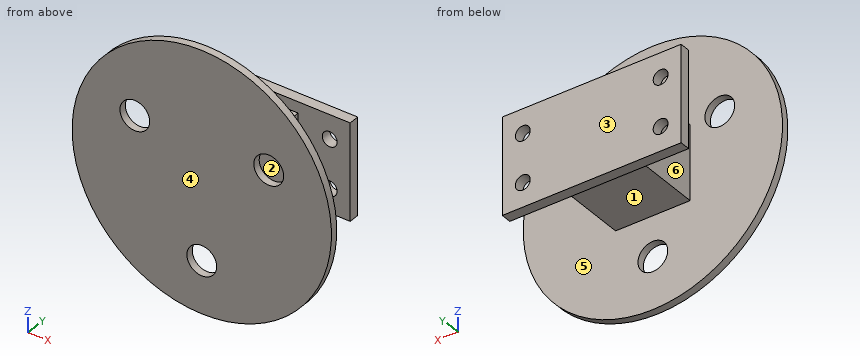
```python
from build123d import *

# Parameters (mm, degrees)
SKETCH1_R           = 87
SKETCH1_R_2         = 10
BOSS_EXTRUDE1_DEPTH = 5
SKETCH2_W           = 50
SKETCH2_H           = 50
BOSS_EXTRUDE2_DEPTH = 50
SKETCH3_W           = 120
SKETCH3_H           = 65
SKETCH3_R           = 5
BOSS_EXTRUDE3_DEPTH = 7


with BuildPart() as part:
    # Sketch1 → Boss-Extrude1 (new body)
    with BuildSketch(Plane(origin=(0, 0, 0), x_dir=(1, 0, 0), z_dir=(0, 1, 0))):
        with Locations(Location((0, 0, 0), (0, 0, 270))):
            Circle(SKETCH1_R)
        with Locations(Location((0, 51.875, 0), (0, 0, 270))):
            Circle(SKETCH1_R_2, mode=Mode.SUBTRACT)
        with Locations(Location((44.926567821, -25.936633975, 0), (0, 0, 270))):
            Circle(SKETCH1_R_2, mode=Mode.SUBTRACT)
        with Locations(Location((-44.923567821, -25.938366025, 0), (0, 0, 270))):
            Circle(SKETCH1_R_2, mode=Mode.SUBTRACT)
    extrude(amount=BOSS_EXTRUDE1_DEPTH)

    # Sketch2 → Boss-Extrude2 (add)
    with BuildSketch(Plane(origin=(0, 5, 0), x_dir=(1, 0, 0), z_dir=(0, 1, 0))):
        Rectangle(SKETCH2_W, SKETCH2_H)
    extrude(amount=BOSS_EXTRUDE2_DEPTH)

    # Sketch3 → Boss-Extrude3 (add)
    with BuildSketch(Plane(origin=(0, 55, 0), x_dir=(1, 0, 0), z_dir=(0, 1, 0))):
        Rectangle(SKETCH3_W, SKETCH3_H)
        with Locations(Location((-46.25, -16.25, 0), (0, 0, 270))):
            Circle(SKETCH3_R, mode=Mode.SUBTRACT)
        with Locations(Location((-46.25, 16.25, 0), (0, 0, 90))):
            Circle(SKETCH3_R, mode=Mode.SUBTRACT)
        with Locations(Location((46.25, -16.25, 0), (0, 0, 90))):
            Circle(SKETCH3_R, mode=Mode.SUBTRACT)
        with Locations(Location((46.25, 16.25, 0), (0, 0, 270))):
            Circle(SKETCH3_R, mode=Mode.SUBTRACT)
    extrude(amount=BOSS_EXTRUDE3_DEPTH)


solid = part.part
```
Can you work these out from the model? Positions are in its coordinate system, mm. Face numbers are marked on the shaded views. A direction names the side the tool comes from. Give positions to 0.01 mm unless a question says otherwise; leave off trailing zeros. Order: outer loops, then holes, each group sorted by start corner. A loop starts at its lowest first (then second) coordinate and runs counter-clockwise, first axis right, second up. Notation, with made-up numbers: (-23, -16) - (34, -16) arc R28 cw to (34, 4) - close; hole circle Ø10 at (-6.75, -32). An arc over 180 degrees is marked (long way). Use a Markdown table: item, result. Add a question column.
Q1. If we section it at B-B on z = -17: Write out the boundary of the cut face in (x, y), plus the area to 3 significant figures.
Q2. Please list where these lines run through material, in increasing order: line 1 along X through (y, z) = (58, 16); line 2 along Z through (x, y) = (-46, 59); line 3 along Y through (x, z) = (-26, 25.5).
Q3. I'm going to push flat-ended pins straight in: pin 1 (12 mm diameter, centred on x = -44.92, z = 25.94, fed in from -Y); pin 2 (23 mm diameter, centred on x = 0, z = -51.875, fed in from +Y); pin 3 (7.5 mm diameter, centred on x = -19, y = 58, fed in from +Z). Where does each tip first touch, or does it pass through?
Q4. If we mould it in two halves opening along Y, with no side actions, what happens to the marked faces 3, 4, 5 and 6? For each: released by +Y, released by -Y, zero draft, split by the parting line, or undercut.
Q5. If we section it at C-C on y = 39.5: Write out the boundary of the cut face in (x, z).
Q6. If we section it at A-A on x = 0: Write out the boundary of the cut face in (y, z) (3 decimals).
Q7. On a 3-axis mill with a long thin cutter (end or side, diameter ignored), from which of +Z, -Z, +X, -X, +Y, -Y can I reach the whole of each face in a straight line? I mean the marked faces 1 and 2. Say none if no direction works.
Answers follow:
| question | item | result |
|---|---|---|
| 1 | outline | (-85.32, 0) - (85.32, 0) - (85.32, 5) - (25, 5) - (25, 55) - (41.31, 55) - (41.31, 62) - (-41.31, 62) - (-41.31, 55) - (-25, 55) - (-25, 5) - (-85.32, 5) - close; (-60, 55) - (-51.19, 55) - (-51.19, 62) - (-60, 62) - close; (51.19, 55) - (60, 55) - (60, 62) - (51.19, 62) - close |
| 1 | area | 4,050 mm^2 |
| 2 | line 1 | x = -60 to -51.24, -41.26 to 41.26, 51.24 to 60 |
| 2 | line 2 | z = -32.5 to -21.24, -11.26 to 11.26, 21.24 to 32.5 |
| 2 | line 3 | y = 0 to 5, 55 to 62 |
| 3 | pin 1 | stops at y = 55 |
| 3 | pin 2 | stops at y = 5 |
| 3 | pin 3 | stops at z = 32.5 |
| 4 | face 3 | released by +Y |
| 4 | face 4 | released by -Y |
| 4 | face 5 | undercut |
| 4 | face 6 | undercut |
| 5 | outline | (-25, -25) - (25, -25) - (25, 25) - (-25, 25) - close |
| 6 | outline | (0, -87) - (5, -87) - (5, -61.875) - (0, -61.875) - close; (0, -41.875) - (5, -41.875) - (5, -25) - (55, -25) - (55, -32.5) - (62, -32.5) - (62, 32.5) - (55, 32.5) - (55, 25) - (5, 25) - (5, 87) - (0, 87) - close |
| 7 | face 1 | -Z, +X, -X |
| 7 | face 2 | +Z, -Z, +X |
